The model under review builds one solid part; all positions refer to its coordinate system, in mm. Face numbers are marked on the shaded views. A direction names the side the tool comes from. Round coordinates to 2 decimals unless told otherwise and drop trailing zeros. Write each loop counter-clockwise with the first axis right and the second up, starting at its lowest first coordinate (ties: lowest second). Pieces come first, ordered by that corner, then holes. Notation, with made-up numbers: (48, 80.5) -> (62, 80.5) arc R25 ccw to (62, 101.5) -> close; hole circle Ø9 at (-17.5, 33.25). An arc over 180 degrees is marked (long way). Return JSON: item names as keys, results as strings. Group by question number.
1. Tool access review of the marked faces 1, 2, 3 and 4: name each direction out of +Z, -Z, +X, -X, +Y, -Y from which nothing blocks a thin tool from reaching the whole face with its end or side.
2. Take a section at C-C, the plane z = 8.25. Give the number of separate pieces and of enclosed holes in the cut face, then the cut area to 3 significant figures.
3. Mouldability with a two-part tool opening along Y and no side actions: class the marked faces 5, 6 and 7 as pulls with the +Y half, pulls with the -Y half, needs draft (parallel to the pull), parting line crosses it, or undercut.
4. Take a section at A-A, the plane y = -8.65. Write out the cut boundary in (x, z).
5. For line 1 along Y through (x, z) = (-14, 8.25); line 2 along Y through (x, z) = (9, 7.5); line 3 along Y through (x, z) = (-11.5, 1.75), list the stretches that pass through material, from the lowest coordinate up. Write a range as from..to.
6. Take a section at B-B, the plane y = 28.35. Write out the cut boundary in (x, z), then the cut area to 3 significant figures.
7. Clearance check with flat-ended pins moving along their axes: P1, Ø6.5, axis at x = -22.12, y = -8.65, coming from the +Z side; P2, Ø1.5, axis at y = -24.5, z = 7.5, coming from the +X side; P3, Ø5, axis at y = -14, z = 7, coming from the -X side; P4, Ø2.5, axis at x = 22.88, y = -34.15, coming from the +Z side. State where each tip first meets the part, or that it passes through.
from build123d import *

# Parameters (mm, degrees)
ESBO_O1_R                = 2
ESBO_O1_R_2              = 4
RESSALTO_EXTRUS_O1_DEPTH = 10
ESBO_O7_W                = 10
ESBO_O7_H                = 15
ESBO_O7_W_2              = 8
ESBO_O7_H_2              = 8
CORTE_EXTRUS_O1_DEPTH    = 55.856129841
CORTE_EXTRUS_O7_DEPTH    = 6
FILETE1_R                = 1
FILETE2_R                = 2


with BuildPart() as part:
    # Esboço1 → Ressalto-extrusão1 (new body)
    with BuildSketch(Plane.XY):
        Polygon((-26.623119185, 32.1), (-26.623119185, 23.6), (-28.123119185, 23.6), (-28.123119185, 7.6), (-26.623119185, 7.6), (-26.623119185, -13.4), (-28.123119185, -13.4), (-28.123119185, -29.4), (-26.623119185, -29.4), (-26.623119185, -37.9), (27.376880815, -37.9), (27.376880815, -29.4), (28.876880815, -29.4), (28.876880815, -13.4), (27.376880815, -13.4), (27.376880815, 7.6), (28.876880815, 7.6), (28.876880815, 23.6), (27.376880815, 23.6), (27.376880815, 32.1), (38.376880815, 32.1), (38.376880815, 37.9), (-37.623119185, 37.9), (-37.623119185, 32.1), align=None)
        with Locations((-22.123119185, 28.35)):
            Circle(ESBO_O1_R, mode=Mode.SUBTRACT)
        with Locations((22.876880815, 28.35)):
            Circle(ESBO_O1_R, mode=Mode.SUBTRACT)
        with Locations((22.876880815, -34.15)):
            Circle(ESBO_O1_R, mode=Mode.SUBTRACT)
        with Locations((-22.123119185, -34.15)):
            Circle(ESBO_O1_R, mode=Mode.SUBTRACT)
        with Locations((-22.123119185, -8.65)):
            Circle(ESBO_O1_R, mode=Mode.SUBTRACT)
        with Locations((22.876880815, -8.65)):
            Circle(ESBO_O1_R, mode=Mode.SUBTRACT)
        with Locations((-22.123119185, 2.85)):
            Circle(ESBO_O1_R, mode=Mode.SUBTRACT)
        with Locations((22.876880815, 2.85)):
            Circle(ESBO_O1_R, mode=Mode.SUBTRACT)
        with Locations((0.376880815, -32.9)):
            Circle(ESBO_O1_R_2, mode=Mode.SUBTRACT)
    extrude(amount=RESSALTO_EXTRUS_O1_DEPTH)

    # Esboço7 → Corte-extrusão1 (cut, through all)
    with BuildSketch(Plane(origin=(0, 0, 0), x_dir=(-1, 0, 0), z_dir=(0, 0, -1))):
        with Locations((14.623119185, -2.9)):
            Rectangle(ESBO_O7_W, ESBO_O7_H)
        with Locations((-0.376880815, 15.6)):
            Rectangle(ESBO_O7_W_2, ESBO_O7_H_2)
        with Locations((-0.376880815, -21.4)):
            Rectangle(ESBO_O7_W_2, ESBO_O7_H_2)
    extrude(amount=-CORTE_EXTRUS_O1_DEPTH, mode=Mode.SUBTRACT)

    # Esboço9 → Corte-extrusão7 (cut)
    with BuildSketch(Plane.XY.offset(10)):
        Polygon((27.376880815, 9.6), (-26.623119185, 9.6), (-26.623119185, 13.6), (-28.623119185, 13.6), (-28.623119185, 17.6), (-26.623119185, 17.6), (-26.623119185, 21.6), (27.376880815, 21.6), (27.376880815, 17.6), (29.376880815, 17.6), (29.376880815, 13.6), (27.376880815, 13.6), align=None)
        Polygon((27.376880815, -15.4), (-26.623119185, -15.4), (-26.623119185, -19.4), (-28.623119185, -19.4), (-28.623119185, -23.4), (-26.623119185, -23.4), (-26.623119185, -27.4), (27.376880815, -27.4), (27.376880815, -23.4), (29.376880815, -23.4), (29.376880815, -19.4), (27.376880815, -19.4), align=None)
    extrude(amount=-CORTE_EXTRUS_O7_DEPTH, mode=Mode.SUBTRACT)

    # Filete1
    filete1_edges = [part.edges().sort_by_distance(p)[0] for p in [
        (28.126880815, 17.6, 4),
        (28.126880815, 13.6, 4),
        (-27.373119185, 13.6, 4),
        (-27.373119185, 17.6, 4),
        (28.126880815, -19.4, 4),
        (28.126880815, -23.4, 4),
        (-27.373119185, -23.4, 4),
        (-27.373119185, -19.4, 4),
    ]]
    fillet(filete1_edges, radius=FILETE1_R)

    # Filete2
    # the kernel refuses this fillet: 2 mm, written as the material it adds along each edge
    with BuildSketch(Plane(origin=(-26.623119185, 23.6, 0), x_dir=(0, 1, 0), z_dir=(0, 0, 1)), Plane(origin=(27.376880815, -29.4, 0), x_dir=(0, -1, 0), z_dir=(0, 0, 1))) as filete2_piece_1:
        with BuildLine():
            CenterArc((1.936491673, 2), FILETE2_R, 194.477512186, 75.522487814)
            Line((0, 1.5), (-0.038729833, 1.49))
            ThreePointArc((-0.038729833, 1.49), (-0.04, 0.75), (-0.04, 0))
            Line((-0.04, 0), (0, -0.04))
            Line((0, -0.04), (1.936491673, -0.04))
            Line((1.936491673, -0.04), (1.936491673, 0))
        make_face()
    extrude(amount=10)
    with BuildSketch(Plane(origin=(27.376880815, 23.6, 0), x_dir=(1, 0, 0), z_dir=(0, 0, 1)), Plane(origin=(-26.623119185, -29.4, 0), x_dir=(-1, 0, 0), z_dir=(0, 0, 1))) as filete2_piece_2:
        with BuildLine():
            CenterArc((2, 1.936491673), FILETE2_R, 180, 75.522487814)
            Line((0, 1.936491673), (-0.04, 1.936491673))
            Line((-0.04, 1.936491673), (-0.04, 0))
            Line((-0.04, 0), (0, -0.04))
            ThreePointArc((0, -0.04), (0.75, -0.04), (1.49, -0.038729833))
            Line((1.49, -0.038729833), (1.5, 0))
        make_face()
    extrude(amount=10)
    with BuildSketch(Plane(origin=(27.376880815, 7.6, 0), x_dir=(1, 0, 0), z_dir=(0, 0, 1)), Plane(origin=(-26.623119185, -13.4, 0), x_dir=(-1, 0, 0), z_dir=(0, 0, 1))) as filete2_piece_3:
        with BuildLine():
            CenterArc((2, -1.936491673), FILETE2_R, 104.477512186, 75.522487814)
            Line((0, -1.936491673), (-0.04, -1.936491673))
            Line((-0.04, -1.936491673), (-0.04, 0))
            Line((-0.04, 0), (0, 0.04))
            ThreePointArc((0, 0.04), (0.75, 0.04), (1.49, 0.038729833))
            Line((1.49, 0.038729833), (1.5, 0))
        make_face()
    extrude(amount=10)
    with BuildSketch(Plane(origin=(27.376880815, -13.4, 0), x_dir=(0, 1, 0), z_dir=(0, 0, 1)), Plane(origin=(-26.623119185, 7.6, 0), x_dir=(0, -1, 0), z_dir=(0, 0, 1))) as filete2_piece_4:
        with BuildLine():
            CenterArc((1.936491673, -2), FILETE2_R, 90, 75.522487814)
            Line((0, -1.5), (-0.038729833, -1.49))
            ThreePointArc((-0.038729833, -1.49), (-0.04, -0.75), (-0.04, 0))
            Line((-0.04, 0), (0, 0.04))
            Line((0, 0.04), (1.936491673, 0.04))
            Line((1.936491673, 0.04), (1.936491673, 0))
        make_face()
    extrude(amount=10)


solid = part.part
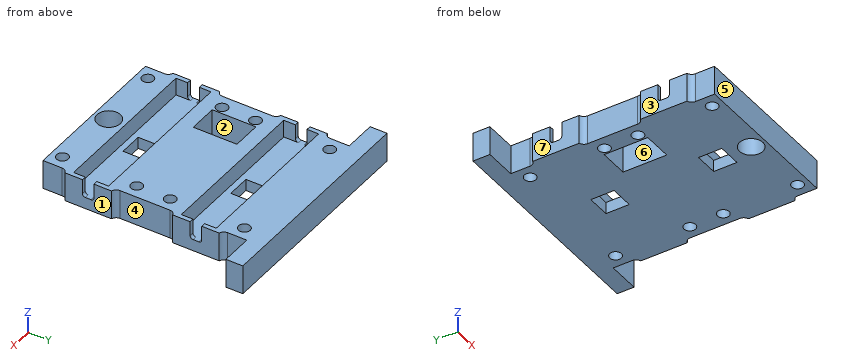
Output:
{
 "1": {"face 1": "+Z, -Z, +X, -Y", "face 2": "+Z, -Z", "face 3": "+Z, -Z, -X, -Y", "face 4": "+Z, -Z, +X"},
 "2": {"separate pieces": "3", "enclosed holes": "10", "area": "2,700 mm^2"},
 "3": {"face 5": "pulls with the -Y half", "face 6": "undercut", "face 7": "needs draft"},
 "4": {"outline": "(-26.62, 0) -> (-24.12, 0) -> (-24.12, 10) -> (-26.62, 10) -> close; (-20.12, 0) -> (-19.62, 0) -> (-19.62, 10) -> (-20.12, 10) -> close; (-9.62, 0) -> (20.88, 0) -> (20.88, 10) -> (-9.62, 10) -> close; (24.88, 0) -> (27.38, 0) -> (27.38, 10) -> (24.88, 10) -> close"},
 "5": {"line 1": "y = -37.9..-27.4, -15.4..-10.4, 4.6..9.6, 21.6..37.9", "line 2": "y = -37.9..-27.4, -15.4..9.6, 21.6..37.9", "line 3": "y = -37.9..-10.4, 4.6..37.9"},
 "6": {"outline": "(-26.62, 0) -> (-24.12, 0) -> (-24.12, 10) -> (-26.62, 10) -> close; (-20.12, 0) -> (20.88, 0) -> (20.88, 10) -> (-20.12, 10) -> close; (24.88, 0) -> (27.38, 0) -> (27.38, 10) -> (24.88, 10) -> close", "area": "460 mm^2"},
 "7": {"P1": "stops at z = 10", "P2": "stops at x = 28.88", "P3": "stops at x = -28.12", "P4": "passes through"}
}
